Source: CAD feature listing. Evaluate the final solid. Frame: model axes, mm. A direction names the side the tool comes from. Coordinates: 2 decimals unless noted, no trailing zeros. Loops run counter-clockwise (first coordinate to the right, second up) from the corner with the lowest first, then second, coordinate; pieces in that order, holes last.
Item 1: Pull-direction query (X, two-part tool) for faces 1 (the flat face through (19.05, -547, -35)), 2 (the flat face through (392, -392, -19.05)), 3 (the flat face through (706.9, -715.5, -25)), 4 (the flat face through (553, 0, -25)); classes: +X half, -X half, draft (parallel to the pull), parting line (faces both ways), or undercut.
Item 2: Section query B-B, the plane x = 319.5. Return the cut outline in (y, z).
Item 3: Section query A-A, the plane z = -39.5. Return the cut outline in (x, y).
Item 4: Section query C-C, the plane y = -595. Return the cut outline in (x, z).
Item 5: Reachability of faces 5 (the flat face through (51.115, -52.026, -34.703)), 6 (the flat face through (280, -16, -50.8)) from +Z, -Z, +X, -X, +Y, -Y: full face, straight path, thin tool, end or side. Return the list, or none.
Item 6: Pin query (flat end, axial travel): pin 1 Ø8 at (y, z) = (-909, -17.5) entering from +X; pin 2 Ø16 at (y, z) = (-476.5, -39.5) entering from +X; pin 3 Ø17 at (x, y) = (939.8, -76.2) entering from -Z; pin 4 Ø16 at (x, z) = (739, -42) entering from -Y. Return the tip coordinate at first contact, or that it passes through.
Item 7: Line query: probe 1 along X at (y, z) = (-207, -34.5); probe 2 along Y at (x, z) = (76, -7); probe 3 along Y at (x, z) = (939.8, -11.75) (3 decimals). Output: solid intervals per line, ascending.
```python
from build123d import *

# Parameters (mm, degrees)
F1_DEPTH = 50.8
F2_DEPTH = 19.05
F3_R     = 9.525
F4_DEPTH = 19.05


with BuildPart() as f1:
    # F0 (on Top) → F1 (new body)
    with BuildSketch(Plane.XY):
        Polygon((0, -76.2), (0, -1016), (406.4, -1016), (1016, -406.4), (1016, 0), (76.2, 0), align=None)
        Polygon((398.509232, -996.95), (19.05, -996.95), (19.05, -84.090768), (84.090768, -19.05), (996.95, -19.05), (996.95, -398.509232), align=None, mode=Mode.SUBTRACT)
    extrude(amount=-F1_DEPTH)

    # F0 (on Top) → F2 (join)
    with BuildSketch(Plane.XY):
        Polygon((19.05, -84.090768), (19.05, -996.95), (398.509232, -996.95), (996.95, -398.509232), (996.95, -19.05), (84.090768, -19.05), align=None)
    extrude(amount=-F2_DEPTH)

    # F3 (on face) → F4 (cut, through all)
    with BuildSketch(Plane(origin=(0, 0, -19.05), x_dir=(1, 0, 0), z_dir=(0, 0, -1))):
        with Locations((76.2, 939.8)):
            Circle(F3_R)
        with Locations((91.981537, 91.981537)):
            Circle(F3_R)
        with Locations((374.836927, 939.8)):
            Circle(F3_R)
        with Locations((939.8, 374.836927)):
            Circle(F3_R)
        with Locations((939.8, 76.2)):
            Circle(F3_R)
    extrude(amount=-F4_DEPTH, mode=Mode.SUBTRACT)


solid = f1.part
```
Verdict:
1. face 1: undercut
1. face 2: undercut
1. face 3: +X half
1. face 4: draft
2. outline: (-1016, -50.8) - (-996.95, -50.8) - (-996.95, -19.05) - (-19.05, -19.05) - (-19.05, -50.8) - (0, -50.8) - (0, 0) - (-1016, 0) - close
3. outline: (0, -1016) - (406.4, -1016) - (1016, -406.4) - (1016, 0) - (76.2, 0) - (0, -76.2) - close; hole (19.05, -996.95) - (398.51, -996.95) - (996.95, -398.51) - (996.95, -19.05) - (84.09, -19.05) - (19.05, -84.09) - close
4. outline: (0, -50.8) - (19.05, -50.8) - (19.05, -19.05) - (800.46, -19.05) - (800.46, -50.8) - (827.4, -50.8) - (827.4, 0) - (0, 0) - close
5. face 5: -Z
5. face 6: -Z, +X, -X, +Y, -Y
6. pin 1: stops at x = 517.4
6. pin 2: stops at x = 953.9
6. pin 3: passes through
6. pin 4: stops at y = -691.4
7. probe 1: x = 0 to 19.05, 996.95 to 1016
7. probe 2: y = -1016 to -949.32, -930.28 to -0.2
7. probe 3: y = -482.6 to -384.362, -365.312 to -85.725, -66.675 to 0
